The drawing under review shows one solid part. Ordinate dimensions are in mm from its lowest x, y, z. Give positions to 0.01 mm unless a question says otherwise; leave off trailing zeros. Order: outer loops, then holes, each group sorted by start corner. A loop starts at its lowest first (then second) coordinate and runs counter-clockwise, first axis right, second up. Notation, with made-up numbers: (3, 75) -> (13, 75) arc R18 cw to (13, 98) -> close; hole circle Ø9 at (88.25, 60.25). An arc over 180 degrees is marked (long way). Use a Markdown table: item, result. Add a question column.
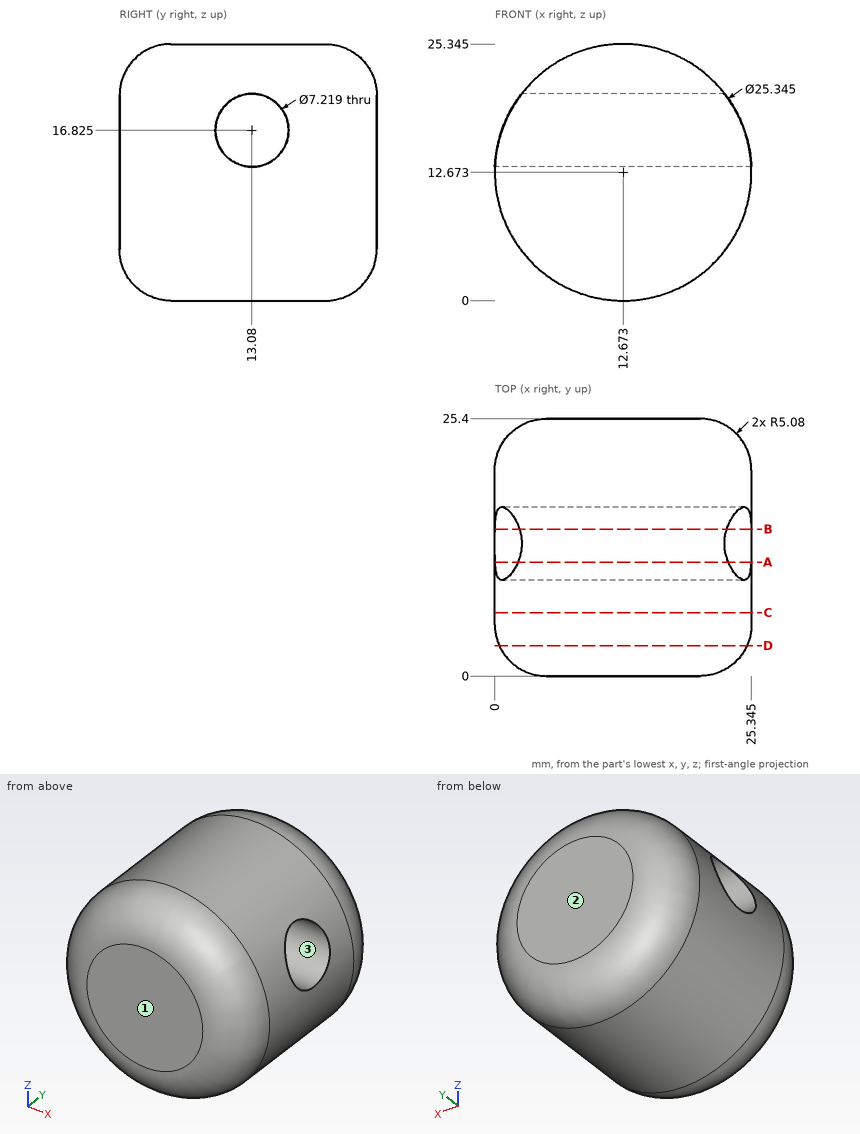
1) Insertion check: pin 1 (6 mm diameter, centred on y = 19, z = 21.5, fed in from +X) (1 decimal); pin 2 (10 mm diameter, centred on y = 19, z = 19.5, fed in from -X); pin 3 (1 mm diameter, centred on x = 3.5, z = 14.5, fed in from -Y). Each pin has a flat end and moves straight along its axis. Give the tip position at first contact, or say it passes through.
2) The part is to be moulded in two halves that separate along Y. For the marked faces 1, 2 and 3, say which applies: +Y half, -Y half, draft (parallel to the pull), parting line (faces both ways), or undercut.
3) Add section D-D (y = 3). Give the boundary of the cut face in (x, z) (1 decimal).
4) Add section A-A (y = 11.25). Give the boundary of the cut face in (x, z) (1 decimal).
5) For L1, parallel to Y at x = 12.5, z = 18; L2, parallel to Z at x = 17.75, y = 13 (1 decimal); L3, parallel to Y at x = 10.25, z = 5.25 (1 decimal), list the stretches that pass through material, from the lowest coordinate up. Write a range as [from, to].
6) Add section C-C (y = 6.25). Give the boundary of the cut face in (x, z) (1 decimal).
7) Add section B-B (y = 14.5). Give the boundary of the cut face in (x, z) (1 decimal).
Worked answers:
| question | item | result |
|---|---|---|
| 1 | pin 1 | x = 23.9 |
| 1 | pin 2 | x = 0.13 |
| 1 | pin 3 | y = 0.16 |
| 2 | face 1 | -Y half |
| 2 | face 2 | +Y half |
| 2 | face 3 | undercut |
| 3 | outline | circle Ø24.5 at (12.7, 12.7) |
| 4 | outline | (0, 13.7) arc R12.7 ccw (long way) to (25.3, 13.7) -> close; (2.3, 19.9) -> (23.1, 19.9) arc R12.7 ccw to start |
| 5 | L1 | [0, 9.67], [16.49, 25.4] |
| 5 | L2 | [1.1, 13.2], [20.4, 24.3] |
| 5 | L3 | [0, 25.4] |
| 6 | outline | circle Ø25.3 at (12.7, 12.7) |
| 7 | outline | (0, 13.5) arc R12.7 ccw (long way) to (25.3, 13.5) -> close; (2.4, 20.1) -> (22.9, 20.1) arc R12.7 ccw to start |
